CAD build for the part. Positions are in the model's coordinates, mm. Round coordinates to 2 decimals unless told otherwise and drop trailing zeros. Loops run counter-clockwise (first coordinate to the right, second up) from the corner with the lowest first, then second, coordinate; pieces in that order, holes last. Notation, with made-up numbers: (34.25, -30.5) - (62.25, -30.5) arc R20 cw to (62.25, -9.5) - close; hole circle Ø9 at (-37, 43.5). An arc over 180 degrees is marked (long way). Use one line per item in the form item = value.
from build123d import *

# Parameters (mm, degrees)
F1_R     = 101.6
F1_R_2   = 4.5494653294
F1_R_3   = 5.1204654318
F1_R_4   = 5.1430144974
F1_R_5   = 5.3478696025
F1_R_6   = 6.3874946109
F3_DEPTH = 25.4


# Not quite as in the source:
# - the program builds the solid bodies; features that only make, move or delete a surface that nothing else refers to are left out


with BuildPart() as f3:
    # F1 (on face) → F3 (new body)
    with BuildSketch(Plane.XZ):
        with Locations((-34.2702679336, 12.4070197344)):
            Circle(F1_R)
        with Locations((-83.0803439021, -27.0566623658)):
            Circle(F1_R_2, mode=Mode.SUBTRACT)
        with Locations((-11.2562878057, -45.9673032165)):
            Circle(F1_R_3, mode=Mode.SUBTRACT)
        with Locations((-87.0806723833, 46.585727483)):
            Circle(F1_R_4, mode=Mode.SUBTRACT)
        with Locations((28.565146029, 15.8559419215)):
            Circle(F1_R_5, mode=Mode.SUBTRACT)
        with Locations((-17.984110862, 72.9515254498)):
            Circle(F1_R_6, mode=Mode.SUBTRACT)
    extrude(amount=F3_DEPTH)


solid = f3.part
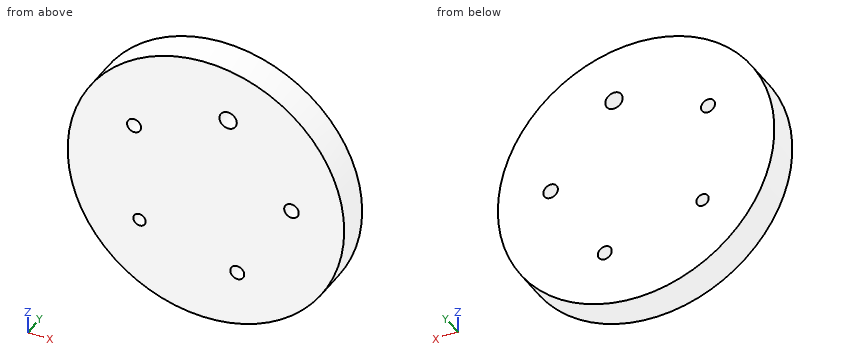
1) Slice it at B-B (z = 100.5). Write the cut outline in (x, y), plus the area to 3 significant figures.
Report:
outline = (-84.89, -25.4) - (16.35, -25.4) - (16.35, 0) - (-84.89, 0) - close
area = 2,570 mm^2
2) Slice it at C-C (x = 8.5). Write the cut outline in (y, z).
Report:
outline = (-25.4, -79.75) - (0, -79.75) - (0, 104.57) - (-25.4, 104.57) - close
3) Slice it at A-A (y = -17.75). Write the cut outline in (x, z).
Report:
outline = circle Ø203.2 at (-34.27, 12.41); hole circle Ø10.29 at (-87.08, 46.59); hole circle Ø9.1 at (-83.08, -27.06); hole circle Ø12.77 at (-17.98, 72.95); hole circle Ø10.24 at (-11.26, -45.97); hole circle Ø10.7 at (28.57, 15.86)
4) Flat gauge pins, fed straight in: pin 1 (1 mm diameter, centred on x = 39, y = -8.5, fed in from +Z); pin 2 (1 mm diameter, centred on y = -12, z = -13.5, fed in from -X); pin 3 (1 mm diameter, centred on y = -4.5, z = 72.5, fed in from +X); pin 4 (2 mm diameter, centred on x = -52.5, z = -60, fed in from +Y). Where does each tip first touch, or does it go through?
Report:
pin_1 = 83.31
pin_2 = -132.64
pin_3 = 48.02
pin_4 = 0
5) Drill centre lines: probe 1 along X at (y, z) = (-1, 45.5); probe 2 along Z at (x, y) = (-11, -16.5); probe 3 along X at (y, z) = (-1.25, -42.5). Where is each one in solid material? Low to high.
Report:
probe_1 = -130.33 to -92.11, -82.05 to 61.79
probe_2 = -86.49 to -51.08, -40.85 to 111.31
probe_3 = -119.76 to -15.02, -7.49 to 51.22
